```python
from build123d import *

# Parameters (mm, degrees)
SKETCH1_W           = 195
SKETCH1_H           = 170
BOSS_EXTRUDE1_DEPTH = 26
SKETCH2_W           = 90
SKETCH2_H           = 20
CUT_EXTRUDE1_DEPTH  = 132.936537775
FILLET1_R           = 15
SKETCH3_W           = 30
SKETCH3_H           = 6
BOSS_EXTRUDE2_DEPTH = 26
CHAMFER1_SIZE       = 20
CHAMFER2_SIZE       = 20
CHAMFER3_SIZE       = 20
SKETCH6_R           = 6.1
CUT_EXTRUDE4_DEPTH  = 3.2
FILLET2_R           = 0.2
CUT_EXTRUDE3_DEPTH  = 23
CUT_EXTRUDE5_DEPTH  = 136.879542242
SKETCH8_W           = 5
SKETCH8_H           = 76.6
BOSS_EXTRUDE3_DEPTH = 7
SKETCH9_W           = 10
SKETCH9_H           = 106.6
CUT_EXTRUDE6_DEPTH  = 5
SKETCH10_W          = 3
SKETCH10_H          = 106.6
CUT_EXTRUDE7_DEPTH  = 20
BOSS_EXTRUDE8_REACH = 166.014
SKETCH14_W          = 6
SKETCH14_H          = 16.5
CUT_EXTRUDE9_DEPTH  = 0.5
SKETCH15_W          = 5
SKETCH15_H          = 23.6
CUT_EXTRUDE10_DEPTH = 10
SKETCH16_W          = 20
SKETCH16_H          = 106.6
CUT_EXTRUDE11_DEPTH = 1


with BuildPart() as part:
    # Sketch1 → Boss-Extrude1 (new body)
    with BuildSketch(Plane(origin=(0, 0, 0), x_dir=(1, 0, 0), z_dir=(0, 1, 0))):
        Rectangle(SKETCH1_W, SKETCH1_H)
    extrude(amount=BOSS_EXTRUDE1_DEPTH)

    # Sketch2 → Cut-Extrude1 (cut, through all)
    with BuildSketch(Plane(origin=(0, 26, 0), x_dir=(1, 0, 0), z_dir=(0, 1, 0))):
        with Locations((-22.5, -75)):
            Rectangle(SKETCH2_W, SKETCH2_H)
        with Locations((-22.5, 75)):
            Rectangle(SKETCH2_W, SKETCH2_H)
    extrude(amount=-CUT_EXTRUDE1_DEPTH, mode=Mode.SUBTRACT)

    # Fillet1
    fillet1_edges = [part.edges().sort_by_distance(p)[0] for p in [
        (-67.5, 13, 65),
        (22.5, 13, 65),
        (-67.5, 13, -65),
        (22.5, 13, -65),
    ]]
    fillet(fillet1_edges, radius=FILLET1_R)

    # Sketch3 → Boss-Extrude2 (add)
    with BuildSketch(Plane(origin=(0, 26, 0), x_dir=(1, 0, 0), z_dir=(0, 1, 0))):
        with Locations((-82.5, 88)):
            Rectangle(SKETCH3_W, SKETCH3_H)
        with Locations((-82.5, -88)):
            Rectangle(SKETCH3_W, SKETCH3_H)
    extrude(amount=-BOSS_EXTRUDE2_DEPTH)

    # Chamfer1
    chamfer1_edges = [part.edges().sort_by_distance(p)[0] for p in [
        (-97.5, 13, -91),
        (-97.5, 13, 91),
    ]]
    chamfer(chamfer1_edges, length=CHAMFER1_SIZE)

    # Chamfer2
    chamfer2_edges = [part.edges().sort_by_distance(p)[0] for p in [
        (-72.5, 26, 91),
        (-72.5, 26, -91),
        (-97.5, 26, 0),
        (-87.5, 26, 81),
        (-87.5, 26, -81),
    ]]
    chamfer(chamfer2_edges, length=CHAMFER2_SIZE)

    # Chamfer3
    chamfer3_edges = [part.edges().sort_by_distance(p)[0] for p in [
        (97.5, 26, 0),
    ]]
    chamfer(chamfer3_edges, length=CHAMFER3_SIZE)

    # Sketch6 → Cut-Extrude4 (cut)
    with BuildSketch(Plane.XZ):
        with Locations(Location((82.166666667, -75, 0), (0, 0, 270))):
            Circle(SKETCH6_R)
        with Locations(Location((82.166666667, 75, 0), (0, 0, 90))):
            Circle(SKETCH6_R)
        with Locations(Location((-75.5, -79.6, 0), (0, 0, 270))):
            Circle(SKETCH6_R)
        with Locations(Location((-75.5, 79.6, 0), (0, 0, 90))):
            Circle(SKETCH6_R)
    extrude(amount=-CUT_EXTRUDE4_DEPTH, mode=Mode.SUBTRACT)

    # Fillet2
    fillet2_edges = [part.edges().sort_by_distance(p)[0] for p in [
        (82.166666667, 0, 68.9),
        (-75.5, 0, -73.5),
        (-75.5, 0, 73.5),
        (82.166666667, 0, -68.9),
    ]]
    fillet(fillet2_edges, radius=FILLET2_R)

    # Sketch5 → Cut-Extrude3 (cut)
    with BuildSketch(Plane.XZ):
        Polygon((-93.5, 38.3), (-77.5, 38.3), (-77.5, 53.3), (-57.5, 53.3), (-57.5, 38.3), (-57.5, -38.3), (-57.5, -53.3), (-77.5, -53.3), (-77.5, -38.3), (-93.5, -38.3), (-96.5, -38.3), (-96.5, -21.8), (-93.5, -21.8), (-77.5, -21.8), (-77.5, 21.8), (-93.5, 21.8), (-96.5, 21.8), (-96.5, 38.3), align=None)
    extrude(amount=-CUT_EXTRUDE3_DEPTH, mode=Mode.SUBTRACT)

    # Sketch7 → Cut-Extrude5 (cut, through all)
    with BuildSketch(Plane.XZ):
        with BuildLine():
            ThreePointArc((-45.328823714, -33.788550396), (-45.093019824, -33.847760063), (-44.855010797, -33.897368154))
            ThreePointArc((-44.855010797, -33.897368154), (-30.428224571, -36.76873565), (-15.749999998, -37.731354711))
            ThreePointArc((-15.749999998, -37.731354711), (14.040735516, -32.512701591), (40.283591791, -17.478249245))
            ThreePointArc((40.283591791, -17.478249245), (48.481354711, 0), (40.283591791, 17.478249245))
            ThreePointArc((40.283591791, 17.478249245), (14.040735515, 32.512701591), (-15.75, 37.731354711))
            ThreePointArc((-15.75, 37.731354711), (-30.428224573, 36.76873565), (-44.855010797, 33.897368153))
            ThreePointArc((-44.855010797, 33.897368153), (-45.093019823, 33.847760063), (-45.328823714, 33.788550395))
            ThreePointArc((-45.328823714, 33.788550395), (-47.992640687, 32.242640687), (-49.538550395, 29.578823714))
            ThreePointArc((-49.538550395, 29.578823714), (-49.597760063, 29.343019823), (-49.647368153, 29.105010797))
            ThreePointArc((-49.647368153, 29.105010797), (-53.481354711, 0), (-49.647368154, -29.105010797))
            ThreePointArc((-49.647368154, -29.105010797), (-49.597760063, -29.343019824), (-49.538550396, -29.578823714))
            ThreePointArc((-49.538550396, -29.578823714), (-47.992640687, -32.242640687), (-45.328823714, -33.788550396))
        make_face()
    extrude(amount=-CUT_EXTRUDE5_DEPTH, mode=Mode.SUBTRACT)

    # Sketch8 → Boss-Extrude3 (add)
    with BuildSketch(Plane.XZ):
        with Locations((-94, 0)):
            Rectangle(SKETCH8_W, SKETCH8_H)
    extrude(amount=-BOSS_EXTRUDE3_DEPTH)

    # Sketch9 → Cut-Extrude6 (cut)
    with BuildSketch(Plane.XZ):
        with Locations((-52.5, 0)):
            Rectangle(SKETCH9_W, SKETCH9_H)
    extrude(amount=-CUT_EXTRUDE6_DEPTH, mode=Mode.SUBTRACT)

    # Sketch10 → Cut-Extrude7 (cut)
    with BuildSketch(Plane.XZ):
        with Locations((-79, 0)):
            Rectangle(SKETCH10_W, SKETCH10_H)
    extrude(amount=-CUT_EXTRUDE7_DEPTH, mode=Mode.SUBTRACT)

    # Boss-Extrude8: up to this face of the body (flat: up to its plane)
    boss_extrude8_end = Plane(part.part.faces().sort_by_distance((-85.605919003, 9.540498442, -38.3))[0])
    # Sketch13 → Boss-Extrude8 (add, up to the picked face)
    with BuildSketch(Plane(origin=(0, 0, 38.3), x_dir=(-1, 0, 0), z_dir=(0, 0, -1)), mode=Mode.PRIVATE) as boss_extrude8_sk1:
        Polygon((80.5, 23), (77.5, 23), (77.5, 22), (81.5, 22), align=None)
    boss_extrude8_tool1 = split(extrude(boss_extrude8_sk1.sketch, amount=BOSS_EXTRUDE8_REACH, mode=Mode.PRIVATE), bisect_by=boss_extrude8_end, keep=Keep.BOTH, mode=Mode.PRIVATE)
    add(boss_extrude8_tool1.solids().sort_by(Axis((-79.261905, 22.47619, 38.3), (0, 0, -1)))[0])

    # Sketch14 → Cut-Extrude9 (cut)
    with BuildSketch(Plane(origin=(0, 7, 0), x_dir=(1, 0, 0), z_dir=(0, 1, 0))):
        with Locations((-94.5, 30.05)):
            Rectangle(SKETCH14_W, SKETCH14_H)
        with Locations((-94.5, -30.05)):
            Rectangle(SKETCH14_W, SKETCH14_H)
    extrude(amount=-CUT_EXTRUDE9_DEPTH, mode=Mode.SUBTRACT)

    # Sketch15 → Cut-Extrude10 (cut)
    with BuildSketch(Plane.XZ):
        with Locations((-83, 0)):
            Rectangle(SKETCH15_W, SKETCH15_H)
    extrude(amount=-CUT_EXTRUDE10_DEPTH, mode=Mode.SUBTRACT)

    # Sketch16 → Cut-Extrude11 (cut)
    with BuildSketch(Plane.XZ.offset(-23)):
        with Locations((-67.5, 0)):
            Rectangle(SKETCH16_W, SKETCH16_H)
    extrude(amount=-CUT_EXTRUDE11_DEPTH, mode=Mode.SUBTRACT)


solid = part.part
```
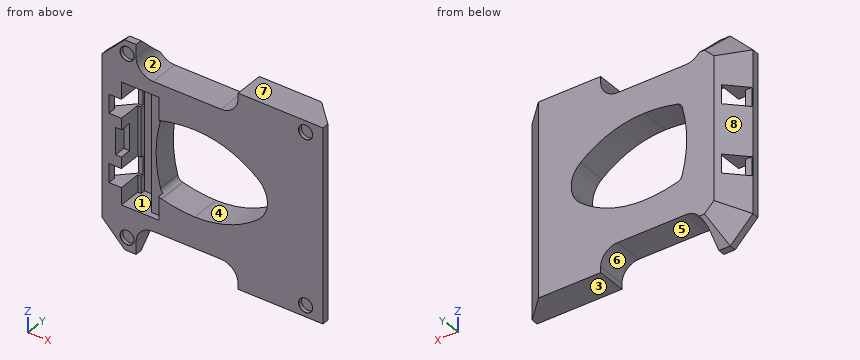
Here's how the part is built. I have some questions about the finished solid (model axes, mm). Face numbers are marked on the shaded views. A direction names the side the tool comes from. Round coordinates to 2 decimals unless told otherwise and drop trailing zeros. Write each loop counter-clockwise with the first axis right and the second up, starting at its lowest first coordinate (ties: lowest second). Pieces come first, ordered by that corner, then holes.
Q1. If we section it at D-D on x = -62: Write out the boundary of the cut face in (y, z), plus the area to 3 significant figures.
Q2. If we mould it in two halves opening along X, with no side actions, what happens to the marked faces 5, 6, 7 and 8? For each: +X half, -X half, draft (parallel to the pull), parting line (faces both ways), or undercut.
Q3. Please list where these lines run through material, in increasing order: probe 1 along Z at (x, y) = (-83.5, 4.75); probe 2 along X at (y, z) = (0.9, -75); probe 3 along Z at (x, y) = (-19, 16).
Q4. If we section it at C-C on y = 13.75: Give the number of separate pieces and of enclosed holes in the cut face, plus the area to 3 significant figures.
Q5. If we section it at A-A on x = -42.5: Write out the boundary of the cut face in (y, z), plus the area to 3 significant figures.
Q6. Will these pins go through, and if not, where does the flat tip stop? P1, Ø8, axis at x = -27, y = 8, coming from the -Z side; P2, Ø1.5, axis at y = 18.5, z = -82.5, coming from the -X side; P3, Ø12, axis at x = 59.5, y = 5.5, coming from the +Z side.
Q7. Which directions (+Z, -Z, +X, -X, +Y, -Y) give clear straight access to the entire face, cutting with the end or side of a thin tool? Please do the marked faces 1, 2, 3 and 4.
Q8. If we section it at B-B on z = -2.5: Write out the boundary of the cut face in (x, y).
Answer below:
1. outline: (0, -68.39) - (26, -68.39) - (26, 68.39) - (0, 68.39) - (0, 53.3) - (24, 53.3) - (24, -53.3) - (0, -53.3) - close
1. area: 998 mm2
2. face 5: undercut
2. face 6: undercut
2. face 7: draft
2. face 8: -X half
3. probe 1: z = -85 to -38.3, -21.8 to -11.8, 11.8 to 21.8, 38.3 to 85
3. probe 2: x = -93.5 to -79.51, -71.49 to -66.64, 21.64 to 76.07, 88.27 to 97.5
3. probe 3: z = -65 to -37.68, 37.68 to 65
4. separate pieces: 2
4. enclosed holes: 1
4. area: 17,700 mm2
5. outline: (0, -65) - (26, -65) - (26, -34.5) - (0, -34.5) - close; (0, 34.5) - (26, 34.5) - (26, 65) - (0, 65) - close
5. area: 1,590 mm2
6. P1: stops at z = -65
6. P2: stops at x = 22.5
6. P3: stops at z = 85
7. face 1: -Y
7. face 2: +Z, +Y, -Y
7. face 3: -Z, +X, +Y, -Y
7. face 4: +Y, -Y
8. outline: (-97.5, 0) - (-85.5, 0) - (-85.5, 10) - (-80.5, 10) - (-80.5, 20) - (-77.5, 20) - (-77.5, 24) - (-57.5, 24) - (-57.5, 5) - (-53.45, 5) - (-53.45, 26) - (-77.5, 26) - (-97.5, 6) - close; (48.34, 0) - (97.5, 0) - (97.5, 6) - (77.5, 26) - (48.34, 26) - close
